Can you work these out from the model? Positions are in its coordinate system, mm. Round coordinates to 2 decimals unless told otherwise and drop trailing zeros. Loops run counter-clockwise (first coordinate to the right, second up) from the corner with the lowest first, then second, coordinate; pieces in that order, holes last.
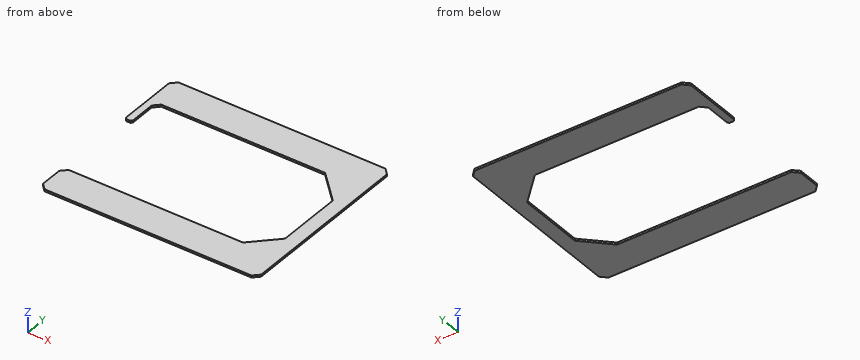
Autodesk Inventor part; units mm, degrees
ref_plane "YZ Plane" through (0, 0, 0) normal (1, 0, 0) x (0, 1, 0)
ref_plane "XZ Plane" through (0, 0, 0) normal (0, 1, 0) x (-1, 0, 0)
ref_plane "XY Plane" through (0, 0, 0) normal (0, 0, 1) x (1, 0, 0)
sketch "Эскиз1" plane through (0, 0, 0) normal (0, 0, 1) x (1, 0, 0)
  line L0 (0, 0) -> (-80.25, 0) construction
  line L1 (-80.25, 0) -> (-80.25, -18.086) construction
  line L2 (-80.25, -18.086) -> (0, -18.086) construction
  line L3 (0, -18.086) -> (0, 0) construction
  line L4 (-80.25, -18.086) -> (-80.25, -42.186) construction
  line L5 (-80.25, -18.086) -> (-56.15, -18.086) construction
  line L6 (-80.25, -42.186) -> (76.75, -42.186)
  line L7 (76.75, -42.186) -> (76.75, 91.214)
  line L8 (76.75, 91.214) -> (-80.25, 91.214)
  line L9 (-80.25, 91.214) -> (-80.25, -42.186)
  line L10 (-80.25, -42.186) -> (76.75, -42.186)
  line L11 (76.75, -42.186) -> (76.75, -18.086)
  line L12 (76.75, -18.086) -> (-80.25, -18.086)
  line L13 (-80.25, -18.086) -> (-80.25, -42.186)
  line L14 (76.75, 91.214) -> (-80.25, 91.214)
  line L15 (-80.25, 91.214) -> (-80.25, 67.114)
  line L16 (-80.25, 67.114) -> (76.75, 67.114)
  line L17 (76.75, 67.114) -> (76.75, 91.214)
  line L18 (-80.25, -42.186) -> (-75.25, -42.186)
  line L19 (-75.25, -42.186) -> (-75.25, 88.814)
  line L20 (-75.25, 88.814) -> (-80.25, 88.814)
  line L21 (-80.25, 88.814) -> (-80.25, -42.186)
  line L22 (76.75, -42.186) -> (66.75, -42.186)
  line L23 (66.75, -42.186) -> (66.75, 88.814)
  line L24 (66.75, 88.814) -> (76.75, 88.814)
  line L25 (76.75, 88.814) -> (76.75, -42.186)
  line L26 (76.75, -42.186) -> (41.75, -42.186)
  line L27 (41.75, -42.186) -> (41.75, -22.186)
  line L28 (41.75, -42.186) -> (61.75, -42.186) construction
  line L29 (76.75, 23.314) -> (-80.25, 23.314)
  line L30 (41.75, 88.814) -> (41.75, 68.814)
  line L31 (66.75, 67.114) -> (66.75, 47.114)
  line L32 (66.75, 47.114) -> (46.75, 67.114)
  line L33 (66.75, 47.114) -> (95.0343, 47.114) construction
  line L34 (66.75, -0.486) -> (46.75, -20.486)
  line L35 (-75.25, 23.314) -> (-80.25, 23.314)
  line L36 (-80.25, 23.314) -> (-80.25, 43.314)
  line L37 (-80.25, 43.314) -> (-75.25, 43.314)
  line L38 (-75.25, 43.314) -> (-75.25, 23.314)
  point P0 (-75.25, -18.086)
  point P1 (-75.25, 67.114)
  point P2 (71.75, 70.413)
  point P3 (66.75, -18.086)
  point P4 (66.75, -0.486)
  point P5 (49.15, -18.086)
  point P6 (-80.25, 43.314)
  point P7 (-75.25, 43.314)
  point P8 (-80.25, -18.086)
  dimension "d0" = 80.25
  dimension "d1" = 18.086
  dimension "d2" = 24.1
  dimension "d3" = 90
  dimension "d4" = 157
  dimension "d5" = 133.4
  dimension "d6" = 157
  dimension "d7" = 24.1
  dimension "d8" = 157
  dimension "d9" = 24.1
  dimension "d10" = 5
  dimension "d11" = 131
  dimension "d12" = 10
  dimension "d13" = 131
  dimension "d16" = 35
  dimension "d17" = 20
  dimension "d18" = 90
  dimension "d19" = 20
  dimension "d20" = 135
  dimension "d21" = 20
extrude "Выдавливание1" add sketch "Эскиз1" along normal blind 1.5 contours L9 L12 L19 L6 | L19 L12 L23 L6 | L23 L12 L7 L6 | L34 L23 L12 | L9 L16 L19 L37 | L23 L29 L7 L12 | L23 L16 L7 L29 | L9 L20 L19 L16 | L19 L20 L9 L8 L7 L24 L23 L16 | L32 L16 L23 | L23 L24 L7 L16
sketch "Эскиз2" plane through (-80.25, -42.186, 0) normal (0, -1, 0) x (1, 0, 0)
  line L0 (129.4, 0) -> (0, 0)
  line L1 (157, 0) -> (0, 0)
  line L2 (0, 0) -> (157, 0)
  line L3 (157, 0) -> (78.5, 0)
  line L4 (78.5, 0) -> (78.5, -20)
  line L5 (78.5, -20) -> (73.5, -20)
  line L6 (73.5, -20) -> (49.6649, 0)
  line L7 (78.5, -20) -> (83.5, -20)
  line L8 (83.5, -20) -> (107.3351, 0)
  point P0 (80.25, 0)
  dimension "d22" = 20
  dimension "d24" = 5
  dimension "d25" = 140
chamfer "Фаска1" distance 4 angle 45 6 edges at (76.75, 91.214, 0.75) (76.75, -42.186, 0.75) (-80.25, -18.086, 0.75) (-80.25, -42.186, 0.75) (-80.25, 91.214, 0.75) (-75.25, 67.114, 0.75)
chamfer "Фаска2" distance 1 angle 45 2 edges at (-80.25, 43.314, 0.75) (-75.25, 43.314, 0.75)
properties part number "sensor board"
(1) If we section it at A-A, the plane x = -55: List the corners of the cut face in (y, z) for me.
Worked answers:
outline: (-42.19, 0) - (-18.09, 0) - (-18.09, 1.5) - (-42.19, 1.5) - close; (67.11, 0) - (91.21, 0) - (91.21, 1.5) - (67.11, 1.5) - close
(2) If I drill on line 1 (Y direction, x = -24, z = 0.55); line 2 (Y direction, x = 63.5, z = 1.4); line 3 (X direction, y = 29.5, z = 0.2), over which ranges is the centre line in solid material (lowest first)?
Worked answers:
line 1: y = -42.19 to -18.09, 67.11 to 91.21
line 2: y = -42.19 to -3.74, 50.36 to 91.21
line 3: x = 66.75 to 76.75
(3) If we section it at B-B, the plane y = 56: List the corners of the cut face in (x, z) for me.
Worked answers:
outline: (-80.25, 0) - (-75.25, 0) - (-75.25, 1.5) - (-80.25, 1.5) - close; (57.86, 0) - (76.75, 0) - (76.75, 1.5) - (57.86, 1.5) - close
(4) If we section it at C-C, the plane z = 0.8: List the corners of the cut face in (x, y) for me, then the cut area to 3 significant figures.
Worked answers:
outline: (-80.25, -38.19) - (-76.25, -42.19) - (72.75, -42.19) - (76.75, -38.19) - (76.75, 87.21) - (72.75, 91.21) - (-76.25, 91.21) - (-80.25, 87.21) - (-80.25, 44.31) - (-79.25, 43.31) - (-76.25, 43.31) - (-75.25, 44.31) - (-75.25, 63.11) - (-71.25, 67.11) - (46.75, 67.11) - (66.75, 47.11) - (66.75, -0.49) - (49.15, -18.09) - (-76.25, -18.09) - (-80.25, -22.09) - close
area: 8,860 mm2
(5) If we section it at D-D, the plane y = 37: List the corners of the cut face in (x, z) for me.
Worked answers:
outline: (66.75, 0) - (76.75, 0) - (76.75, 1.5) - (66.75, 1.5) - close
